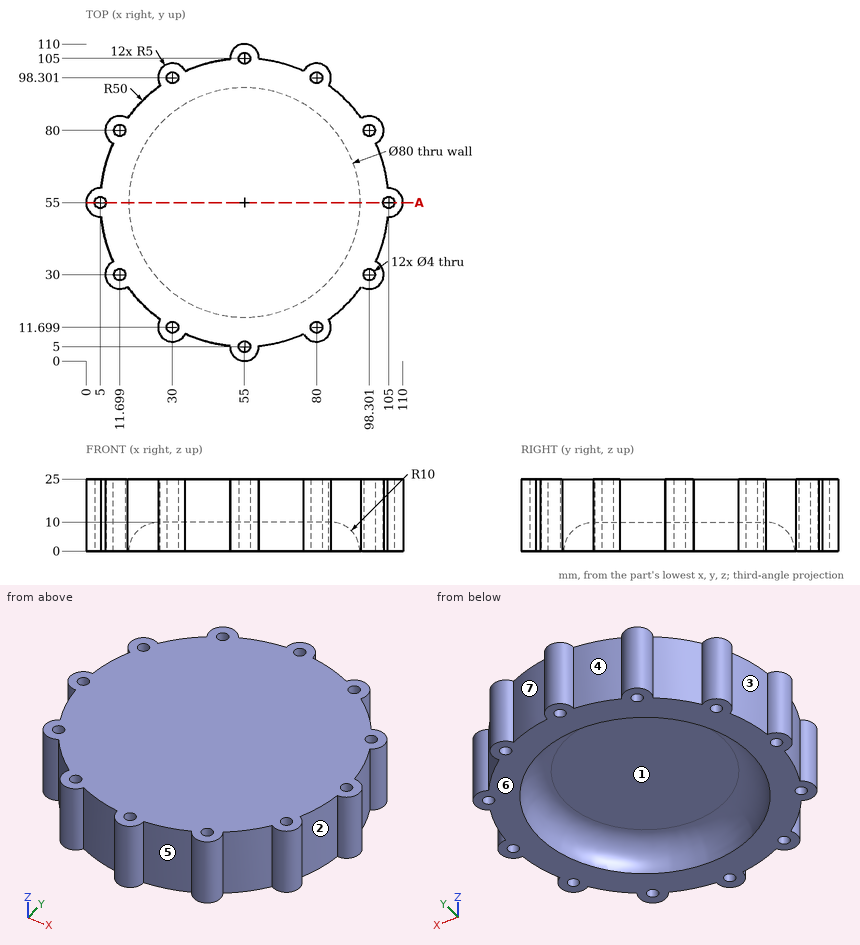
Drawing for the job (mm, zero at the part's lowest x, y, z). A direction names the side the tool comes from. Give positions to 0.01 mm unless a question says otherwise; leave off trailing zeros. Write item = value, one per line. Start each with the question number.
1. Cut at A-A, the plane y = 55. State how many separate pieces and enclosed holes the cut face has, and give its area (3 significant figures).
2. Which spindle directions (+Z, -Z, +X, -X, +Y, -Y) get a long thin tool onto all of the face, cutting with end or side? Do the marked faces 5, 6 and 7. Say none if no direction does.
3. Two-plate mould, pull along X, no slides. Class the marked faces 1, 2, 3 and 4: pulls with the +X half, pulls with the -X half, needs draft (parallel to the pull), parting line crosses it, or undercut.
4. Probe line 1 along Y through (x, z) = (55, 10.5); line 2 along Y through (x, z) = (11.5, 6.75); line 3 along Z through (x, y) = (50, 28). List the from-to ranges inside material, lowest first.
5. Drop flat-ended pins along their axis: P1, Ø4, axis at y = 14, z = 13.5, coming from the -X side; P2, Ø4.5, axis at x = 55, y = 5, coming from the -Z side; P3, Ø3, axis at y = 77, z = 6.5, coming from the +X side; P4, Ø1.5, axis at y = 14.5, z = 17, coming from the -X side. Give the stop position or say it passes through.
Taken from the geometry:
q1.separate_pieces = 3
q1.enclosed_holes = 0
q1.area = 1,790 mm²
q2.face_5 = +Z, -Z, -Y
q2.face_6 = -Z, +X, -X, +Y, -Y
q2.face_7 = +Z, -Z, +Y
q3.face_1 = undercut
q3.face_2 = pulls with the +X half
q3.face_3 = pulls with the -X half
q3.face_4 = undercut
q4.line_1 = 0 to 3, 7 to 103, 107 to 110
q4.line_2 = 25 to 28.01, 31.99 to 78.01, 81.99 to 85
q4.line_3 = 10 to 25
q5.P1 = 23.71
q5.P2 = 0
q5.P3 = 103.07
q5.P4 = 24.67
